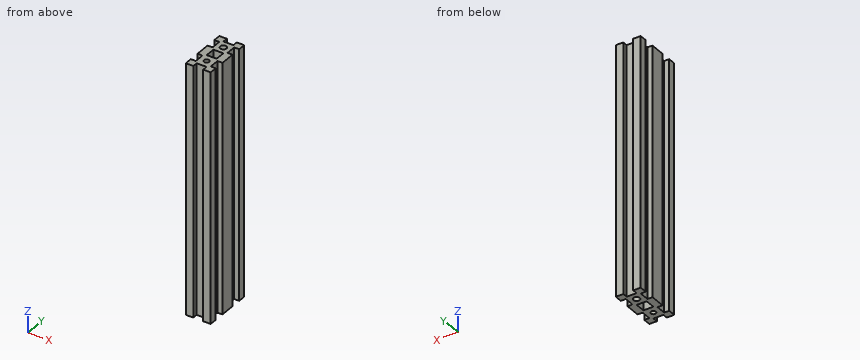
Autodesk Inventor part; units mm, degrees
ref_plane "YZ Plane" through (0, 0, 0) normal (1, 0, 0) x (0, 1, 0)
ref_plane "XZ Plane" through (0, 0, 0) normal (0, 1, 0) x (-1, 0, 0)
ref_plane "XY Plane" through (0, 0, 0) normal (0, 0, 1) x (1, 0, 0)
sketch "Sketch1" plane through (0, 0, 0) normal (0, 0, 1) x (1, 0, 0)
  line L0 (10, -10) -> (-10, 10) construction
  line L1 (-10, -10) -> (10, 10) construction
  line L2 (-4, 6) -> (4, 6)
  line L3 (4, 6) -> (4, 14)
  line L4 (4, 14) -> (-4, 14)
  line L5 (-4, 14) -> (-4, 6)
  line L6 (-4, 6) -> (4, 14) construction
  line L7 (4, 6) -> (-4, 14) construction
  line L8 (14, -4) -> (6, -4)
  line L9 (6, -4) -> (6, 4)
  line L10 (6, 4) -> (14, 4)
  line L11 (14, 4) -> (14, -4)
  line L12 (14, -4) -> (6, 4) construction
  line L13 (6, -4) -> (14, 4) construction
  line L14 (-4, -6) -> (4, -6)
  line L15 (4, -6) -> (4, -14)
  line L16 (4, -14) -> (-4, -14)
  line L17 (-4, -14) -> (-4, -6)
  line L18 (-4, -6) -> (4, -14) construction
  line L19 (4, -6) -> (-4, -14) construction
  line L20 (-14, 4) -> (-6, 4)
  line L21 (-6, 4) -> (-6, -4)
  line L22 (-6, -4) -> (-14, -4)
  line L23 (-14, -4) -> (-14, 4)
  line L24 (-14, 4) -> (-6, -4) construction
  line L25 (-6, 4) -> (-14, -4) construction
  line L26 (-10, -10) -> (-10, 0)
  line L27 (-10, 4) -> (-10, 10)
  line L28 (-10, 10) -> (0, 10)
  line L29 (4, 10) -> (10, 10)
  line L30 (10, 10) -> (10, 4)
  line L31 (10, 0) -> (10, -10)
  line L32 (10, -10) -> (4, -10)
  line L33 (0, -10) -> (-10, -10)
  point P0 (0, 0)
  point P1 (-4, 10)
  point P2 (10, -4)
  point P3 (-4, -10)
  point P4 (-10, -4)
  dimension "d0" = 20
  dimension "d1" = 20
  dimension "d2" = 8
  dimension "d3" = 8
  dimension "d4" = 8
  dimension "d5" = 8
  dimension "d6" = 8
  dimension "d7" = 8
  dimension "d8" = 8
  dimension "d9" = 8
extrude "Extrusion1" add sketch "Sketch1" along normal blind 200 contours L2 L3 L29 L30 L10 L9 L8 L31 L32 L15 L14 L17 L33 L26 L22 L21 L20 L27 L28 L5
ref_plane "Work Plane1" through (4, 0, 0) normal (0, 1, 0) x (1, 0, 0)
ref_plane "Work Plane2" through (0, -10, 0) normal (1, 0, 0) x (0, 0, -1)
mirror "Mirror1" about plane through (10, 10, 0) normal (0, 1, 0) of "Extrusion1"
sketch "Sketch2" plane through (0, 0, 200) normal (0, 0, 1) x (1, 0, 0)
  line L0 (-10, 4) -> (-10, 16)
  line L1 (-10, 4) -> (-6, 4)
  line L2 (-6, 4) -> (-6, -4)
  line L3 (-6, -4) -> (-10, -4)
  line L4 (-10, -4) -> (-10, -10)
  line L5 (-10, -10) -> (-4, -10)
  line L6 (-4, -10) -> (-4, -6)
  line L7 (-4, -6) -> (4, -6)
  line L8 (4, -6) -> (4, -10)
  line L9 (4, -10) -> (10, -10)
  line L10 (10, -10) -> (10, -4)
  line L11 (10, -4) -> (6, -4)
  line L12 (6, -4) -> (6, 4)
  line L13 (6, 4) -> (10, 4)
  line L14 (10, 4) -> (10, 16)
  line L15 (6, 16) -> (10, 16)
  line L16 (6, 24) -> (6, 16)
  line L17 (10, 24) -> (6, 24)
  line L18 (10, 30) -> (10, 24)
  line L19 (4, 30) -> (10, 30)
  line L20 (4, 26) -> (4, 30)
  line L21 (-4, 26) -> (4, 26)
  line L22 (-4, 30) -> (-4, 26)
  line L23 (-10, 30) -> (-4, 30)
  line L24 (-10, 24) -> (-10, 30)
  line L25 (-6, 24) -> (-10, 24)
  line L26 (-6, 16) -> (-6, 24)
  line L27 (-10, 16) -> (-6, 16)
  line L28 (-4, 6) -> (-4, 14)
  line L29 (4, 14) -> (-4, 14)
  line L30 (4, 6) -> (4, 14)
  line L31 (4, 6) -> (-4, 6)
  circle A0 centre (0, 20) radius 2.5
  circle A1 centre (0, 0) radius 2
  point P0 (0, 0)
  dimension "d12" = 5
  dimension "d13" = 4
  dimension "d14" = 20
  dimension "d15" = 10
extrude "Extrusion2" cut sketch "Sketch2" against normal through all contours A0 | A1
ref_plane "Work Plane3" through (0, 4, 200) normal (1, 0, 0) x (0, 0, -1)
properties part number "Neje_Base_Rod_20mm"
Check sheet for the modelled part. Datum: model origin and axes. Units: mm. Round coordinates to 2 decimals unless told otherwise and drop trailing zeros. Loops run counter-clockwise (first coordinate to the right, second up) from the corner with the lowest first, then second, coordinate; pieces in that order, holes last.
1. Sectioned sample at A-A on y = 9. Record the boundary of the cut face in (x, z), and give its area (3 significant figures).
2. Scan lines: probe 1 along Y at (x, z) = (0, 159.5); probe 2 along Y at (x, z) = (-9, 121); probe 3 along Y at (x, z) = (0.5, 21). Record each from-to range of solid material in increasing order.
3. Sectioned sample at D-D on x = 0. Record the boundary of the cut face in (y, z).
4. Gauge pin test, flat end, axial feed: pin 1 Ø4 at (x, z) = (0, 62.5) entering from +Y. Record the tip position at first contact, or that the pin passes through.
5. Sectioned sample at C-C on z = 74. Give the number of separate pieces and of enclosed holes in the cut face, and give its area (3 significant figures).
6. Sectioned sample at B-B on x = -8.25. Record the boundary of the cut face in (y, z), and give its area (3 significant figures).
Recorded:
1. outline: (-10, 0) - (-4, 0) - (-4, 200) - (-10, 200) - close; (4, 0) - (10, 0) - (10, 200) - (4, 200) - close
1. area: 2,400 mm2
2. probe 1: y = -6 to -2, 2 to 6, 14 to 17.5, 22.5 to 26
2. probe 2: y = -10 to -4, 4 to 16, 24 to 30
2. probe 3: y = -6 to -1.94, 1.94 to 6, 14 to 17.55, 22.45 to 26
3. outline: (-6, 0) - (-2, 0) - (-2, 200) - (-6, 200) - close; (2, 0) - (6, 0) - (6, 200) - (2, 200) - close; (14, 0) - (17.5, 0) - (17.5, 200) - (14, 200) - close; (22.5, 0) - (26, 0) - (26, 200) - (22.5, 200) - close
4. pin 1: stops at y = 26
5. separate pieces: 1
5. enclosed holes: 3
5. area: 512 mm2
6. outline: (-10, 0) - (-4, 0) - (-4, 200) - (-10, 200) - close; (4, 0) - (16, 0) - (16, 200) - (4, 200) - close; (24, 0) - (30, 0) - (30, 200) - (24, 200) - close
6. area: 4,800 mm2
